Design review of the part built by this model. Coordinates are the model's own, in mm. Face numbers are marked on the shaded views. A direction names the side the tool comes from. Give positions to 0.01 mm unless a question says otherwise; leave off trailing zeros. Write each loop counter-clockwise with the first axis right and the second up, starting at its lowest first coordinate (ties: lowest second). Pieces come first, ordered by that corner, then holes.
```python
from build123d import *

# Parameters (mm, degrees)
SKETCH2_R           = 2
BOSS_EXTRUDE1_DEPTH = 17.06
SKETCH3_R           = 1.5
BOSS_EXTRUDE2_DEPTH = 12
SKETCH4_W           = 3.988125856
SKETCH4_H           = 4
BOSS_EXTRUDE3_DEPTH = 2
SKETCH5_W           = 2
SKETCH5_H           = 4
BOSS_EXTRUDE4_DEPTH = 19
FILLET1_R           = 2
FILLET2_R           = 2
FILLET3_R           = 2
SKETCH6_R           = 1.5
CUT_EXTRUDE1_DEPTH  = 34.726600777
SKETCH10_W          = 8
SKETCH10_H          = 2
BOSS_EXTRUDE8_DEPTH = 17.06
FILLET6_R           = 2


with BuildPart() as part:
    # Sketch2 → Boss-Extrude1 (new body)
    with BuildSketch(Plane(origin=(0, 0, 0), x_dir=(0, 0, -1), z_dir=(1, 0, 0))):
        Circle(SKETCH2_R)
    extrude(amount=BOSS_EXTRUDE1_DEPTH)

    # Sketch3 → Boss-Extrude2 (add)
    with BuildSketch(Plane(origin=(17.06, 0, 0), x_dir=(0, 0, -1), z_dir=(1, 0, 0))):
        Circle(SKETCH3_R)
    extrude(amount=BOSS_EXTRUDE2_DEPTH)

    # Sketch4 → Boss-Extrude3 (add)
    with BuildSketch(Plane(origin=(29.06, 0, 0), x_dir=(0, 0, -1), z_dir=(1, 0, 0))):
        with Locations((-0.005937072, 0)):
            Rectangle(SKETCH4_W, SKETCH4_H)
    extrude(amount=-BOSS_EXTRUDE3_DEPTH)

    # Sketch5 → Boss-Extrude4 (add)
    with BuildSketch(Plane.XY.offset(2)):
        with Locations((28.06, 0)):
            Rectangle(SKETCH5_W, SKETCH5_H)
    extrude(amount=-BOSS_EXTRUDE4_DEPTH)

    # Fillet1
    fillet1_edges = [part.edges().sort_by_distance(p)[0] for p in [
        (28.06, 2, 2),
    ]]
    fillet(fillet1_edges, radius=FILLET1_R)

    # Fillet2
    fillet2_edges = [part.edges().sort_by_distance(p)[0] for p in [
        (28.06, -2, 2),
    ]]
    fillet(fillet2_edges, radius=FILLET2_R - 0.0001)  # a hair under: the kernel refuses the full size

    # Fillet3
    fillet3_edges = [part.edges().sort_by_distance(p)[0] for p in [
        (28.06, -2, -17),
        (28.06, 2, -17),
    ]]
    fillet(fillet3_edges, radius=FILLET3_R - 0.0001)  # a hair under: the kernel refuses the full size

    # Sketch6 → Cut-Extrude1 (cut, through all)
    with BuildSketch(Plane(origin=(29.06, 0, 0), x_dir=(0, 0, -1), z_dir=(1, 0, 0))):
        with Locations((15, 0)):
            Circle(SKETCH6_R)
    extrude(amount=-CUT_EXTRUDE1_DEPTH, mode=Mode.SUBTRACT)

    # Sketch10 → Boss-Extrude8 (add)
    with BuildSketch(Plane.ZY):
        with Locations((4, 1)):
            Rectangle(SKETCH10_W, SKETCH10_H)
    extrude(amount=-BOSS_EXTRUDE8_DEPTH)

    # Fillet6
    fillet6_edges = [part.edges().sort_by_distance(p)[0] for p in [
        (8.53, 2, 8),
    ]]
    fillet(fillet6_edges, radius=FILLET6_R - 0.0001)  # a hair under: the kernel refuses the full size


solid = part.part
```
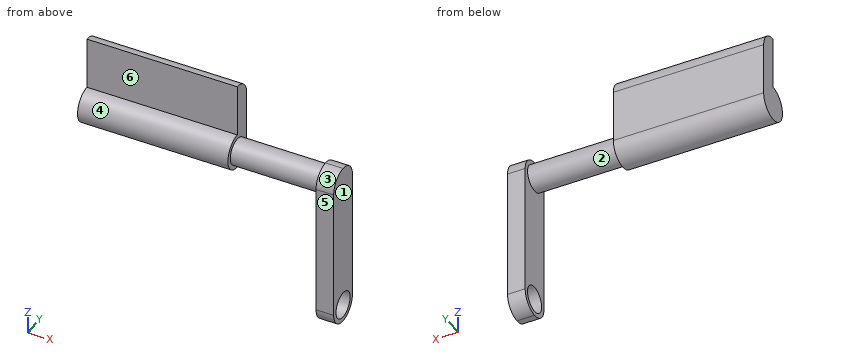
(1) Mouldability with a two-part tool opening along X and no side actions: class the marked faces 1, 2 and 3 as pulls with the +X half, pulls with the -X half, needs draft (parallel to the pull), parting line crosses it, or undercut.
Resolved:
face 1: pulls with the +X half
face 2: undercut
face 3: needs draft
(2) Consider section C-C, the plane x = 25. Give the boundary of the cut face in (y, z).
Resolved:
outline: circle Ø3 at (0, 0)
(3) Consider section B-B, the plane z = 6.5. Give the boundary of the cut face in (x, y).
Resolved:
outline: (0, 0) - (17.06, 0) - (17.06, 1.94) - (0, 1.94) - close
(4) Tool access review of the marked faces 4, 5 and 6: name each direction out of +Z, -Z, +X, -X, +Y, -Y from which nothing blocks a thin tool from reaching the whole face with its end or side.
Resolved:
face 4: -X
face 5: +Z, -Z, +X, -X, -Y
face 6: +Z, +X, -X, -Y
(5) To check wall thickness, follow L1, parallel to X at y = 1.6, z = -0.5; L2, parallel to Y at x = 28.1, z = -15; L3, parallel to X at y = 1.5, z = -11. State the ranges of each line that lie inside material, in increasing order.
Resolved:
L1: x = 0 to 17.06, 27.06 to 29.06
L2: y = -2 to -1.5, 1.5 to 2
L3: x = 27.06 to 29.06
(6) Clearance check with flat-ended pins moving along their axes: P1, Ø1.2, axis at y = 0, z = -5, coming from the -X side; P2, Ø2, axis at x = 19, y = -1, coming from the +Z side; P3, Ø2, axis at y = 1, z = 5, coming from the +X side. State where each tip first meets the part, or that it passes through.
Resolved:
P1: stops at x = 27.06
P2: stops at z = 1.5
P3: stops at x = 17.06
